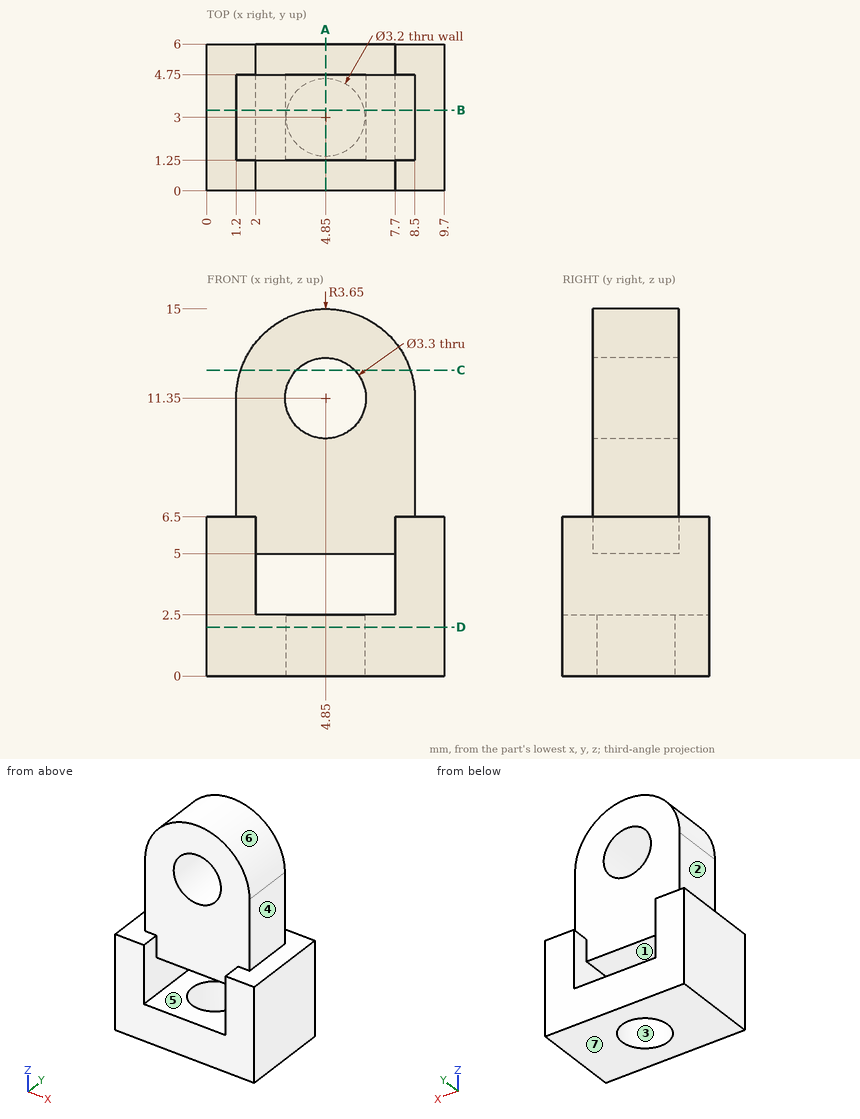
Can you work these out from the drawing? Everything is in mm from the part's minimum corner. A direction names the side the tool comes from. Give positions to 0.01 mm unless a question says otherwise; leave off trailing zeros. Loops run counter-clockwise (first coordinate to the right, second up) from the corner with the lowest first, then second, coordinate; pieces in that order, holes last. Notation, with made-up numbers: (-5, -32.5) - (12, -32.5) arc R4 cw to (12, -25.5) - close; hole circle Ø5 at (39, 62). An arc over 180 degrees is marked (long way). Use one line per item in the form item = value.
1. Thinking about a two-plate mould opening in Z: for the marked faces 4, 5, 6 and 7, which applies, released by +Z, released by -Z, zero draft, split by the parting line, or undercut?
Response values:
face_4 = zero draft
face_5 = undercut
face_6 = released by +Z
face_7 = released by -Z
2. I'm going to push flat-ended pins straight in: pin 1 Ø0.6 at (x, y) = (1.5, 3) entering from +Z (3 decimals); pin 2 Ø3.5 at (x, z) = (3.5, 8.5) entering from +Y; pin 3 Ø1.8 at (y, z) = (3.5, 9) entering from +X. Where does each tip first touch, or does it pass through?
Response values:
pin_1 = 13.355
pin_2 = 4.75
pin_3 = 8.5
3. I want a section at D-D (z = 2). Please give me the cut outline in (x, y), and give its area (3 significant figures).
Response values:
outline = (0, 0) - (9.7, 0) - (9.7, 6) - (0, 6) - close; hole circle Ø3.2 at (4.85, 3)
area = 50.2 mm²
4. I want a section at B-B (y = 3.3). Please give me the cut outline in (x, z).
Response values:
outline = (0, 0) - (3.28, 0) - (3.28, 2.5) - (2, 2.5) - (2, 5) - (7.7, 5) - (7.7, 2.5) - (6.42, 2.5) - (6.42, 0) - (9.7, 0) - (9.7, 6.5) - (8.5, 6.5) - (8.5, 11.35) arc R3.65 ccw to (1.2, 11.35) - (1.2, 6.5) - (0, 6.5) - close; hole circle Ø3.3 at (4.85, 11.35)
5. On a 3-axis mill with a long thin cutter (end or side, diameter ignored), from which of +Z, -Z, +X, -X, +Y, -Y can I reach the whole of each face in a straight line? I mean the marked faces 1, 2 and 3. Say none if no direction works.
Response values:
face_1 = +Y, -Y
face_2 = +Z, -X, +Y, -Y
face_3 = -Z
6. I need wall thicknesses on probe 1 along Y at (x, z) = (4.85, 0.6); probe 2 along Z at (x, y) = (0.5, 5.4); probe 3 along Y at (x, z) = (3.5, 6.25). Which ranges of each line are inside material? Lowest first, please.
Response values:
probe_1 = 0 to 1.4, 4.6 to 6
probe_2 = 0 to 6.5
probe_3 = 1.25 to 4.75
7. I want a section at C-C (z = 12.5). Please give me the cut outline in (x, y), and give its area (3 significant figures).
Response values:
outline = (1.39, 1.25) - (3.67, 1.25) - (3.67, 4.75) - (1.39, 4.75) - close; (6.03, 1.25) - (8.31, 1.25) - (8.31, 4.75) - (6.03, 4.75) - close
area = 16.0 mm²
8. I want a section at A-A (x = 4.85). Please give me the cut outline in (y, z), and give its area (4 significant figures).
Response values:
outline = (0, 0) - (1.4, 0) - (1.4, 2.5) - (0, 2.5) - close; (1.25, 5) - (4.75, 5) - (4.75, 9.7) - (1.25, 9.7) - close; (1.25, 13) - (4.75, 13) - (4.75, 15) - (1.25, 15) - close; (4.6, 0) - (6, 0) - (6, 2.5) - (4.6, 2.5) - close
area = 30.45 mm²
